Geometry check sheet. Reference: the model listing, model coordinates, mm. A direction names the side the tool comes from. Give positions to 0.01 mm unless a question says otherwise; leave off trailing zeros. Write each loop counter-clockwise with the first axis right and the second up, starting at its lowest first coordinate (ties: lowest second). Pieces come first, ordered by that corner, then holes. Notation, with made-up numbers: (20.5, 84.25) - (46.5, 84.25) arc R11 cw to (46.5, 94.25) - close; hole circle Ø6 at (53.25, 71). An arc over 180 degrees is marked (long way). Write item = value, one per line. Start each with the question number.
(1) Section check A-A, the plane x = 0. Enter the section's corners in (y, z), plus the area to 3 significant figures.
(2) Draft check along X on faces 3 (the flat face through (75, 74, 0)), 4 (the flat face through (80, 150, 0)), 5 (the flat face through (85, 71, 0)). Enter one of: pulls with the +X half, pulls with the -X half, needs draft (parallel to the pull), parting line crosses it, or undercut.
(3) Access from +Z, -Z, +X, -X, +Y, -Y to the whole of each face (thin tool, end or side, straight path). Record for faces 1 (the flat face through (-80, 150, 0)), 2 (the flat face through (-75, 76, 0)).
(4) Section check C-C, the plane z = 0. Enter the section's corners in (x, y), plus the area to 3 significant figures.
(5) Section check B-B, the plane y = 120. Enter the section's corners in (x, z).
(6) Section check D-D, the plane y = 72.5. Enter the section's corners in (x, z), plus the area to 3 significant figures.
(7) Thickness scan on L1, parallel to X at y = 39, z = 6.5; L2, parallel to Z at x = 0, y = -4; L3, parallel to X at y = -2, z = 0. Record the ranges inside material, lowest first.
(8) Depth check by flat-ended pin: pin 1 Ø16 at (y, z) = (120, 0) entering from -X; pin 2 Ø6 at (x, z) = (39, -12) entering from +Y. Enter the tip coordinate at first touch or a pass-through.
```python
from build123d import *

# Parameters (mm, degrees)
BOSS_EXTRUDE1_DEPTH     = 30
CUT_EXTRUDE1_DEPTH      = 229.691932521
CUT_EXTRUDE1_DEPTH_BACK = 229.691932521
SKETCH2_R               = 10
CUT_EXTRUDE2_DEPTH      = 184.643676722
CUT_EXTRUDE2_DEPTH_BACK = 184.643676722
SKETCH3_R               = 10


with BuildPart() as part:
    # Sketch1 → Boss-Extrude1 (new, symmetric)
    with BuildSketch(Plane.XY):
        Polygon((0, 0), (75, 0), (75, 150), (85, 150), (85, -10), (0, -10), (-85, -10), (-85, 150), (-75, 150), (-75, 0), align=None)
    extrude(amount=BOSS_EXTRUDE1_DEPTH, both=True)

    # Sketch2 → Cut-Extrude1 (cut, two sides: drawn at the far end of the back side and taken through both)
    with BuildSketch(Plane(origin=(85, 0, 0), x_dir=(0, 0, -1), z_dir=(1, 0, 0)).offset(-CUT_EXTRUDE1_DEPTH_BACK)):
        with Locations((0, 120)):
            Circle(SKETCH2_R)
    extrude(amount=CUT_EXTRUDE1_DEPTH + CUT_EXTRUDE1_DEPTH_BACK, mode=Mode.SUBTRACT)

    # Sketch3 → Cut-Extrude2 (cut, two sides: drawn at the far end of the back side and taken through both)
    with BuildSketch(Plane.XZ.offset(10).offset(-CUT_EXTRUDE2_DEPTH_BACK)):
        with Locations(Location((0, 0, 0), (0, 0, 270))):
            Circle(SKETCH3_R)
    extrude(amount=CUT_EXTRUDE2_DEPTH + CUT_EXTRUDE2_DEPTH_BACK, mode=Mode.SUBTRACT)


solid = part.part
```
Model answer:
q1.outline = (-10, -30) - (0, -30) - (0, -10) - (-10, -10) - close; (-10, 10) - (0, 10) - (0, 30) - (-10, 30) - close
q1.area = 400 mm²
q2.face_3 = undercut
q2.face_4 = needs draft
q2.face_5 = pulls with the +X half
q3.face_1 = +Z, -Z, +X, -X, +Y
q3.face_2 = +Z, -Z, +Y
q4.outline = (-85, -10) - (-10, -10) - (-10, 0) - (-75, 0) - (-75, 110) - (-85, 110) - close; (-85, 130) - (-75, 130) - (-75, 150) - (-85, 150) - close; (10, -10) - (85, -10) - (85, 110) - (75, 110) - (75, 0) - (10, 0) - close; (75, 130) - (85, 130) - (85, 150) - (75, 150) - close
q4.area = 4,100 mm²
q5.outline = (-85, -30) - (-75, -30) - (-75, -10) - (-85, -10) - close; (-85, 10) - (-75, 10) - (-75, 30) - (-85, 30) - close; (75, -30) - (85, -30) - (85, -10) - (75, -10) - close; (75, 10) - (85, 10) - (85, 30) - (75, 30) - close
q6.outline = (-85, -30) - (-75, -30) - (-75, 30) - (-85, 30) - close; (75, -30) - (85, -30) - (85, 30) - (75, 30) - close
q6.area = 1,200 mm²
q7.L1 = -85 to -75, 75 to 85
q7.L2 = -30 to -10, 10 to 30
q7.L3 = -85 to -10, 10 to 85
q8.pin_1 = through
q8.pin_2 = 0
